Input: part model. Units: mm. Frame: model coordinates. Face numbers are marked on the shaded views. A direction names the side the tool comes from. Coordinates: 2 decimals unless noted, no trailing zeros. Order: outer loops, then holes, each group sorted by start corner. A loop starts at its lowest first (then second) coordinate and runs counter-clockwise, first axis right, second up. Notation, with made-up numbers: (77.25, -10) -> (127.25, -10) arc R34 cw to (127.25, 23) -> close; hole circle Ø8 at (-20, 58.5). An arc over 180 degrees is marked (long way). Answer as CSV lines item,"result".
from build123d import *

# Parameters (mm, degrees)
F1_DEPTH = 76.2


with BuildPart() as f1:
    # F0 (on Front) → F1 (new body)
    with BuildSketch(Plane.XZ):
        Polygon((-38.1, 25.4), (-76.2, 25.4), (-76.2, -25.4), (-38.1, -25.4), (-50.8, -8.636308), (50.8, -8.636308), (38.1, -25.4), (76.2, -25.4), (76.2, 25.4), (38.1, 25.4), align=None)
        Polygon((-50.8, 42.153515), (-38.1, 25.4), (38.1, 25.4), (50.8, 42.153515), align=None)
    extrude(amount=F1_DEPTH)


solid = f1.part
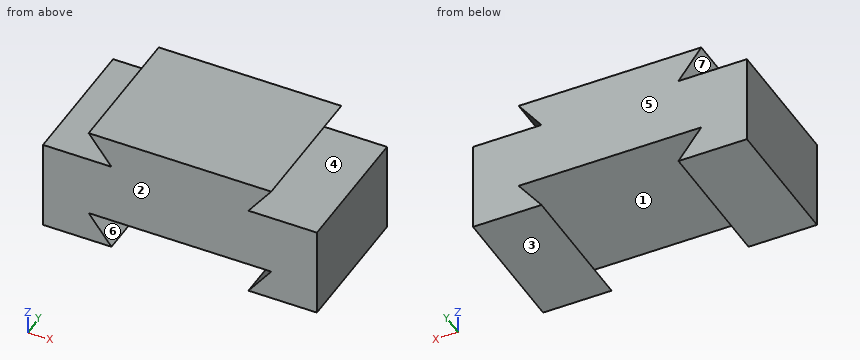
1. Mould query, pull axis Z, two halves, no side actions, for the marked faces 1, 2 and 3. Classes: released by +Z, released by -Z, zero draft, split by the parting line, or undercut.
Findings:
face 1,"undercut"
face 2,"zero draft"
face 3,"released by -Z"
2. Cut plane B-B (x = 58.5). Return the cut outline in (y, z), plus the area to 3 significant figures.
Findings:
outline,"(-76.2, -25.4) -> (0, -25.4) -> (0, 25.4) -> (-76.2, 25.4) -> close"
area,"3,870 mm2"
3. Contact query for a flat-ended pin moving along its axis: pin 1 (23 mm diameter, centred on x = -17, y = -27.5, fed in from -Z). Output: stop coordinate, or through.
Findings:
pin 1,"stops at z = -8.64"
4. Ray query, line 1 along Z through (x, y) = (-49, -39); line 2 along Z through (x, y) = (-45, -47.5); line 3 along Z through (x, y) = (51, -42). Return the intervals inside material, ascending.
Findings:
line 1,"z = -25.4 to -11.01, -8.64 to 25.4, 39.78 to 42.15"
line 2,"z = -25.4 to -16.29, -8.64 to 25.4, 34.5 to 42.15"
line 3,"z = -25.4 to 25.4"
5. Cut plane A-A (y = -64). Return the cut outline in (x, z).
Findings:
outline,"(-76.2, -25.4) -> (-38.1, -25.4) -> (-50.8, -8.64) -> (50.8, -8.64) -> (38.1, -25.4) -> (76.2, -25.4) -> (76.2, 25.4) -> (38.1, 25.4) -> (50.8, 42.15) -> (-50.8, 42.15) -> (-38.1, 25.4) -> (-76.2, 25.4) -> close"
6. Reachability of the marked faces 4, 5, 6 and 7 from +Z, -Z, +X, -X, +Y, -Y: full face, straight path, thin tool, end or side. Return the list, or none.
Findings:
face 4,"+X, +Y, -Y"
face 5,"+Z, -Z, +X, -X, +Y"
face 6,"+Y, -Y"
face 7,"-X, +Y, -Y"
7. Cut plane C-C (x = 4). Return the cut outline in (y, z), plus the area to 3 significant figures.
Findings:
outline,"(-76.2, -8.64) -> (0, -8.64) -> (0, 42.15) -> (-76.2, 42.15) -> close"
area,"3,870 mm2"
